Geometry check sheet. Reference: drawing and pictorial views, mm from the part's lowest x, y, z. A direction names the side the tool comes from. Round coordinates to 2 decimals unless told otherwise and drop trailing zeros. Order: outer loops, then holes, each group sorted by start corner. A loop starts at its lowest first (then second) coordinate and runs counter-clockwise, first axis right, second up.
(1) Release check for a two-part mould opening along X. For the marked faces 1, 2 and 3 record: +X half, -X half, draft (parallel to the pull), parting line (faces both ways), or undercut.
(2) Go/stop test with flat-tipped pins: pin 1 (3 mm diameter, centred on x = 47.5, z = 22, fed in from -Y); pin 2 (4 mm diameter, centred on x = 127.5, z = 9, fed in from +Y); pin 3 (1.5 mm diameter, centred on y = 31, z = 19, fed in from +X); pin 4 (5.5 mm diameter, centred on y = 31, z = 19.5, fed in from -X). Record where each tip stops, or that it passes through.
(3) Set-up check for the marked faces 4 and 5: record each of +Z, -Z, +X, -X, +Y, -Y from which the full face is reachable in a straight line by a thin tool's end or side.
(4) Sectioned sample at D-D (z = 14.5). Record the boundary of the cut face in (x, y).
(5) Sectioned sample at C-C (x = 17). Record the boundary of the cut face in (y, z), plus the area to 3 significant figures.
(6) Material ranges on line 1 along Z through (x, y) = (127.5, 6.25); line 2 along Z through (x, y) = (40, 21.5); line 3 along X through (y, z) = (13, 16), recorded low to high.
(7) Sectioned sample at A-A (z = 9). Give the number of separate pieces and of enclosed holes in the cut face, plus the area to 3 significant figures.
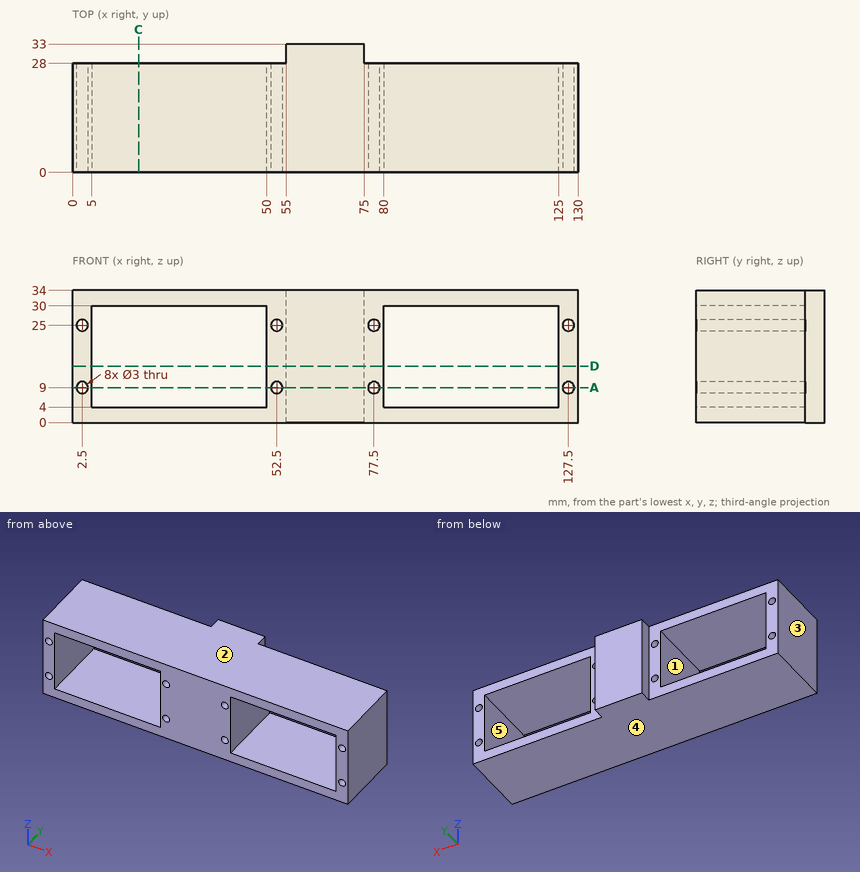
Answer below:
1. face 1: undercut
1. face 2: draft
1. face 3: -X half
2. pin 1: passes through
2. pin 2: stops at y = 28
2. pin 3: stops at x = 75
2. pin 4: stops at x = 55
3. face 4: -Z, +X, -X, +Y, -Y
3. face 5: +Y, -Y
4. outline: (0, 0) - (5, 0) - (5, 28) - (0, 28) - close; (50, 0) - (80, 0) - (80, 28) - (75, 28) - (75, 33) - (55, 33) - (55, 28) - (50, 28) - close; (125, 0) - (130, 0) - (130, 28) - (125, 28) - close
5. outline: (0, 0) - (28, 0) - (28, 4) - (0, 4) - close; (0, 30) - (28, 30) - (28, 34) - (0, 34) - close
5. area: 224 mm2
6. line 1: z = 0 to 7.5, 10.5 to 23.5, 26.5 to 34
6. line 2: z = 0 to 4, 30 to 34
6. line 3: x = 0 to 5, 50 to 80, 125 to 130
7. separate pieces: 7
7. enclosed holes: 0
7. area: 884 mm2
